Read the model definition and answer for the solid it produces. Units are mm, in the model's axes. A direction names the side the tool comes from. Coordinates: 2 decimals unless noted, no trailing zeros. Write each loop counter-clockwise with the first axis right and the second up, starting at its lowest first coordinate (ties: lowest second). Pieces come first, ordered by that corner, then holes. Notation, with made-up numbers: (-14.5, 66.5) -> (16.5, 66.5) arc R21 cw to (16.5, 94.5) -> close; hole circle Ø2 at (-34, 43.25). An arc over 180 degrees is marked (long way). Answer as a JSON object with one key per item and string values. Group by question number.
(1) Find section C-C (y = 1). Give the vertices of the cut face in (x, z).
(2) Flat-ended cylindrical pins translate along their axes: P1, Ø6, axis at x = -3, y = 16.5, coming from the +Z side; P2, Ø10, axis at x = -10.5, y = 11, coming from the +Z side; P3, Ø10.5, axis at x = -5, z = -5, coming from the +Y side; P4, Ø6, axis at x = -10, y = 5.5, coming from the +Z side. Find the tip coordinate at first contact, or state that the pin passes through.
(3) Straight lines are drawn through the part: L1, parallel to X at y = 12.5, z = 0; L2, parallel to Z at x = 4, y = 16; L3, parallel to X at y = 18.75, z = -5. For each, find the intervals that lie inside material, in ascending order.
(4) For a pull along X with two mould halves and no side action, classify faces 1 (the face through (14.415, -0.021, -12.534)), 2 (the face through (16.93, -0.02, -16.9)), 3 (the face through (0, 0, 17.5)) as +X half, -X half, draft (parallel to the pull), parting line (faces both ways), or undercut.
(5) Which of the six approach directions +Z, -Z, +X, -X, +Y, -Y give full straight-line access (tool end or side, diameter ignored) to faces 4 (the face through (-16.93, -0.02, -16.9)), 5 (the face through (-12, 1.5, -8))?
(6) Find section B-B (z = 0). Give the vertices of the cut face in (x, y), then the cut area to 3 significant figures.
(7) Find section D-D (y = 9.5). Give the vertices of the cut face in (x, z), then the cut area to 3 significant figures.
(8) Find section A-A (x = 0). Give the vertices of the cut face in (y, z), then the cut area to 3 significant figures.
from build123d import *

# Parameters (mm, degrees)
ESBO_O1_W                = 35
ESBO_O1_H                = 35
ESBO_O1_R                = 10
ESBO_O1_R_2              = 1.5
RESSALTO_EXTRUS_O1_DEPTH = 1.5
FILETE1_R                = 2
ESBO_O2_R                = 11.5
ESBO_O2_R_2              = 10
RESSALTO_EXTRUS_O2_DEPTH = 23
FILETE2_R                = 2


with BuildPart() as part:
    # Esboço1 → Ressalto-extrusão1 (new, symmetric)
    with BuildSketch(Plane(origin=(0, 0, 0), x_dir=(1, 0, 0), z_dir=(0, 1, 0))):
        Rectangle(ESBO_O1_W, ESBO_O1_H)
        with Locations(Location((0, 0, 0), (0, 0, 270))):
            Circle(ESBO_O1_R, mode=Mode.SUBTRACT)
        with Locations(Location((-13.964466094, 13.964466094, 0), (0, 0, 270))):
            Circle(ESBO_O1_R_2, mode=Mode.SUBTRACT)
        with Locations(Location((13.964466094, 13.964466094, 0), (0, 0, 270))):
            Circle(ESBO_O1_R_2, mode=Mode.SUBTRACT)
        with Locations(Location((13.964466094, -13.964466094, 0), (0, 0, 270))):
            Circle(ESBO_O1_R_2, mode=Mode.SUBTRACT)
        with Locations(Location((-13.964466094, -13.964466094, 0), (0, 0, 270))):
            Circle(ESBO_O1_R_2, mode=Mode.SUBTRACT)
    extrude(amount=RESSALTO_EXTRUS_O1_DEPTH, both=True)

    # Filete1
    filete1_edges = [part.edges().sort_by_distance(p)[0] for p in [
        (17.5, 0, 17.5),
        (-17.5, 0, 17.5),
        (-17.5, 0, -17.5),
        (17.5, 0, -17.5),
    ]]
    fillet(filete1_edges, radius=FILETE1_R)

    # Esboço2 → Ressalto-extrusão2 (add)
    with BuildSketch(Plane(origin=(0, 1.5, 0), x_dir=(1, 0, 0), z_dir=(0, 1, 0))):
        with Locations(Location((0, 0, 0), (0, 0, 90))):
            Circle(ESBO_O2_R)
        with Locations(Location((0, 0, 0), (0, 0, 270))):
            Circle(ESBO_O2_R_2, mode=Mode.SUBTRACT)
    extrude(amount=RESSALTO_EXTRUS_O2_DEPTH)

    # Filete2
    # the kernel refuses this fillet: 2 mm, written as the material it adds along each edge
    with BuildSketch(Plane(origin=(0, 1.5, 0), x_dir=(0, 0, -1), z_dir=(1, 0, 0))) as filete2_piece_1:
        with BuildLine():
            CenterArc((11.5 + FILETE2_R, FILETE2_R), FILETE2_R, 180, 90)
            Line((11.5, FILETE2_R), (11.5, 0))
            Line((11.5, 0), (11.5 + FILETE2_R, 0))
        make_face()
    revolve(axis=Axis((0, 1.5, 0), (0, 1, 0)))
    # the kernel refuses this fillet: 2 mm, written as the material it takes off along each edge
    with BuildSketch(Plane(origin=(0, 24.5, 0), x_dir=(0, 0, -1), z_dir=(1, 0, 0))) as filete2_2_piece_1:
        with BuildLine():
            CenterArc((9.5, -1.936491673), FILETE2_R, 0, 75.522487814)
            Line((11.5, -1.936491673), (11.5, 0))
            Line((11.5, 0), (10, 0))
        make_face()
    revolve(axis=Axis((0, 24.5, 0), (0, 1, 0)), mode=Mode.SUBTRACT)


solid = part.part
Results below:
{
 "1": {"outline": "(-17.5, -15.5) arc R2 ccw to (-15.5, -17.5) -> (15.5, -17.5) arc R2 ccw to (17.5, -15.5) -> (17.5, 15.5) arc R2 ccw to (15.5, 17.5) -> (-15.5, 17.5) arc R2 ccw to (-17.5, 15.5) -> close; hole circle Ø3 at (-13.96, -13.96); hole circle Ø3 at (-13.96, 13.96); hole circle Ø20 at (0, 0); hole circle Ø3 at (13.96, -13.96); hole circle Ø3 at (13.96, 13.96)"},
 "2": {"P1": "stops at z = 11.5", "P2": "stops at z = 10.1", "P3": "stops at y = 24.5", "P4": "stops at z = 9.12"},
 "3": {"L1": "x = -11.5 to -10, 10 to 11.5", "L2": "z = -10.78 to -9.17, 9.17 to 10.78", "L3": "x = -10.36 to -8.66, 8.66 to 10.36"},
 "4": {"face 1": "undercut", "face 2": "+X half", "face 3": "draft"},
 "5": {"face 4": "-Z, -X, +Y, -Y", "face 5": "+Y"},
 "6": {"outline": "(-17.5, -1.5) -> (-10, -1.5) -> (-10, 24.5) arc R2 ccw to (-11.5, 22.56) -> (-11.5, 3.5) arc R2 cw to (-13.5, 1.5) -> (-17.5, 1.5) -> close; (10, -1.5) -> (17.5, -1.5) -> (17.5, 1.5) -> (13.5, 1.5) arc R2 cw to (11.5, 3.5) -> (11.5, 22.56) arc R2 ccw to (10, 24.5) -> close", "area": "114 mm2"},
 "7": {"outline": "circle Ø23 at (0, 0); hole circle Ø20 at (0, 0)", "area": "101 mm2"},
 "8": {"outline": "(-1.5, -17.5) -> (1.5, -17.5) -> (1.5, -13.5) arc R2 cw to (3.5, -11.5) -> (22.56, -11.5) arc R2 ccw to (24.5, -10) -> (-1.5, -10) -> close; (-1.5, 10) -> (24.5, 10) arc R2 ccw to (22.56, 11.5) -> (3.5, 11.5) arc R2 cw to (1.5, 13.5) -> (1.5, 17.5) -> (-1.5, 17.5) -> close", "area": "114 mm2"}
}
